Autodesk Inventor part; units mm, degrees
ref_plane "YZ Plane" through (0, 0, 0) normal (1, 0, 0) x (0, 1, 0)
ref_plane "XZ Plane" through (0, 0, 0) normal (0, 1, 0) x (-1, 0, 0)
ref_plane "XY Plane" through (0, 0, 0) normal (0, 0, 1) x (1, 0, 0)
sketch "Sketch1" plane through (0, 0, 0) normal (0, 0, 1) x (1, 0, 0)
  arc A0 (11.6951, -1.7956) -> (0, 0) centre (4.624, -8.8667) ccw
  line L0 (11.6951, -1.7956) -> (21.2005, -11.301)
  arc A1 (21.2005, -11.301) -> (22.9683, -12.0332) centre (22.9683, -9.5332) ccw
  line L1 (22.9683, -12.0332) -> (26.5038, -12.0332)
  arc A2 (26.5038, -12.0332) -> (29.0038, -9.5332) centre (26.5038, -9.5332) ccw
  line L2 (29.0038, -9.5332) -> (29.0038, -5.9977)
  arc A3 (29.0038, -5.9977) -> (28.2716, -4.2299) centre (26.5038, -5.9977) ccw
  line L3 (28.2716, -4.2299) -> (18.7662, 5.2754)
  arc A4 (16.9706, 16.9706) -> (18.7662, 5.2754) centre (25.8373, 12.3465) ccw
  arc A5 (16.9706, 16.9706) -> (16.9706, 53.963) centre (-18.4962, 35.4668) ccw
  arc A6 (18.7662, 65.6581) -> (16.9706, 53.963) centre (25.8373, 58.587) ccw
  line L4 (18.7662, 65.6581) -> (28.2716, 75.1635)
  arc A7 (28.2716, 75.1635) -> (29.0038, 76.9312) centre (26.5038, 76.9312) ccw
  line L5 (29.0038, 76.9312) -> (29.0038, 80.4668)
  arc A8 (29.0038, 80.4668) -> (26.5038, 82.9668) centre (26.5038, 80.4668) ccw
  line L6 (26.5038, 82.9668) -> (22.9683, 82.9668)
  arc A9 (22.9683, 82.9668) -> (21.2005, 82.2345) centre (22.9683, 80.4668) ccw
  line L7 (21.2005, 82.2345) -> (11.6951, 72.7291)
  arc A10 (0, 70.9335) -> (11.6951, 72.7291) centre (4.624, 79.8002) ccw
  arc A11 (0, 70.9335) -> (-36.9924, 70.9335) centre (-18.4962, 35.4668) ccw
  arc A12 (-48.6875, 72.7291) -> (-36.9924, 70.9335) centre (-41.6164, 79.8002) ccw
  line L8 (-48.6875, 72.7291) -> (-58.1929, 82.2345)
  arc A13 (-58.1929, 82.2345) -> (-59.9607, 82.9668) centre (-59.9607, 80.4668) ccw
  line L9 (-59.9607, 82.9668) -> (-63.4962, 82.9668)
  arc A14 (-63.4962, 82.9668) -> (-65.9962, 80.4668) centre (-63.4962, 80.4668) ccw
  line L10 (-65.9962, 80.4668) -> (-65.9962, 76.9312)
  arc A15 (-65.9962, 76.9312) -> (-65.264, 75.1635) centre (-63.4962, 76.9312) ccw
  line L11 (-65.264, 75.1635) -> (-55.7586, 65.6581)
  arc A16 (-53.9629, 53.963) -> (-55.7586, 65.6581) centre (-62.8296, 58.587) ccw
  arc A17 (-53.9629, 53.963) -> (-53.963, 16.9706) centre (-18.4962, 35.4668) ccw
  arc A18 (-55.7586, 5.2754) -> (-53.963, 16.9706) centre (-62.8296, 12.3465) ccw
  line L12 (-55.7586, 5.2754) -> (-65.264, -4.2299)
  arc A19 (-65.264, -4.2299) -> (-65.9962, -5.9977) centre (-63.4962, -5.9977) ccw
  line L13 (-65.9962, -5.9977) -> (-65.9962, -9.5332)
  arc A20 (-65.9962, -9.5332) -> (-63.4962, -12.0332) centre (-63.4962, -9.5332) ccw
  line L14 (-63.4962, -12.0332) -> (-59.9607, -12.0332)
  arc A21 (-59.9607, -12.0332) -> (-58.1929, -11.301) centre (-59.9607, -9.5332) ccw
  line L15 (-58.1929, -11.301) -> (-48.6875, -1.7956)
  arc A22 (-36.9924, 0) -> (-48.6875, -1.7956) centre (-41.6164, -8.8667) ccw
  arc A23 (-36.9924, 0) -> (-18.9962, -4.5301) centre (-18.4962, 35.4668) ccw
  arc A24 (-18.9962, -4.5301) -> (-17.9962, -4.5301) centre (-18.4962, -4.5332) ccw
  arc A25 (-17.9962, -4.5301) -> (0, 0) centre (-18.4962, 35.4668) ccw
  circle A26 centre (-49.9962, 3.9668) radius 3
  circle A27 centre (-49.9962, 66.9668) radius 3
  circle A28 centre (13.0038, 3.9668) radius 3
  circle A29 centre (13.0038, 66.9668) radius 3
  circle A30 centre (-18.4962, 35.4668) radius 36
extrude "Extrusion1" add sketch "Sketch1" along normal blind 400
sketch "Sketch2" plane through (0, 0, 400) normal (0, 0, 1) x (1, 0, 0)
  circle A0 centre (-18.4962, 35.4668) radius 36
  circle A1 centre (13.0038, 66.9668) radius 3
  circle A2 centre (13.0038, 3.9668) radius 3
  circle A3 centre (-49.9962, 66.9668) radius 3
  circle A4 centre (-49.9962, 3.9668) radius 3
  arc A5 (-17.9962, -4.5301) -> (0, 0) centre (-18.4962, 35.4668) ccw
  arc A6 (11.6951, -1.7956) -> (0, 0) centre (4.624, -8.8667) ccw
  line L0 (21.2005, -11.301) -> (11.6951, -1.7956)
  arc A7 (21.2005, -11.301) -> (22.9683, -12.0332) centre (22.9683, -9.5332) ccw
  line L1 (26.5038, -12.0332) -> (22.9683, -12.0332)
  arc A8 (26.5038, -12.0332) -> (29.0038, -9.5332) centre (26.5038, -9.5332) ccw
  line L2 (29.0038, -5.9977) -> (29.0038, -9.5332)
  arc A9 (29.0038, -5.9977) -> (28.2716, -4.2299) centre (26.5038, -5.9977) ccw
  line L3 (18.7662, 5.2754) -> (28.2716, -4.2299)
  arc A10 (16.9706, 16.9706) -> (18.7662, 5.2754) centre (25.8373, 12.3465) ccw
  arc A11 (16.9706, 16.9706) -> (16.9706, 53.963) centre (-18.4962, 35.4668) ccw
  arc A12 (18.7662, 65.6581) -> (16.9706, 53.963) centre (25.8373, 58.587) ccw
  line L4 (28.2716, 75.1635) -> (18.7662, 65.6581)
  arc A13 (28.2716, 75.1635) -> (29.0038, 76.9312) centre (26.5038, 76.9312) ccw
  line L5 (29.0038, 80.4668) -> (29.0038, 76.9312)
  arc A14 (29.0038, 80.4668) -> (26.5038, 82.9668) centre (26.5038, 80.4668) ccw
  line L6 (22.9683, 82.9668) -> (26.5038, 82.9668)
  arc A15 (22.9683, 82.9668) -> (21.2005, 82.2345) centre (22.9683, 80.4668) ccw
  line L7 (11.6951, 72.7291) -> (21.2005, 82.2345)
  arc A16 (0, 70.9335) -> (11.6951, 72.7291) centre (4.624, 79.8002) ccw
  arc A17 (0, 70.9335) -> (-36.9924, 70.9335) centre (-18.4962, 35.4668) ccw
  arc A18 (-48.6875, 72.7291) -> (-36.9924, 70.9335) centre (-41.6164, 79.8002) ccw
  line L8 (-58.1929, 82.2345) -> (-48.6875, 72.7291)
  arc A19 (-58.1929, 82.2345) -> (-59.9607, 82.9668) centre (-59.9607, 80.4668) ccw
  line L9 (-63.4962, 82.9668) -> (-59.9607, 82.9668)
  arc A20 (-63.4962, 82.9668) -> (-65.9962, 80.4668) centre (-63.4962, 80.4668) ccw
  line L10 (-65.9962, 76.9312) -> (-65.9962, 80.4668)
  arc A21 (-65.9962, 76.9312) -> (-65.264, 75.1635) centre (-63.4962, 76.9312) ccw
  line L11 (-55.7586, 65.6581) -> (-65.264, 75.1635)
  arc A22 (-53.9629, 53.963) -> (-55.7586, 65.6581) centre (-62.8296, 58.587) ccw
  arc A23 (-53.9629, 53.963) -> (-53.963, 16.9706) centre (-18.4962, 35.4668) ccw
  arc A24 (-55.7586, 5.2754) -> (-53.963, 16.9706) centre (-62.8296, 12.3465) ccw
  line L12 (-65.264, -4.2299) -> (-55.7586, 5.2754)
  arc A25 (-65.264, -4.2299) -> (-65.9962, -5.9977) centre (-63.4962, -5.9977) ccw
  line L13 (-65.9962, -9.5332) -> (-65.9962, -5.9977)
  arc A26 (-65.9962, -9.5332) -> (-63.4962, -12.0332) centre (-63.4962, -9.5332) ccw
  line L14 (-59.9607, -12.0332) -> (-63.4962, -12.0332)
  arc A27 (-59.9607, -12.0332) -> (-58.1929, -11.301) centre (-59.9607, -9.5332) ccw
  line L15 (-48.6875, -1.7956) -> (-58.1929, -11.301)
  arc A28 (-36.9924, 0) -> (-48.6875, -1.7956) centre (-41.6164, -8.8667) ccw
  arc A29 (-36.9924, 0) -> (-18.9962, -4.5301) centre (-18.4962, 35.4668) ccw
  arc A30 (-18.9962, -4.5301) -> (-17.9962, -4.5301) centre (-18.4962, -4.5332) ccw
extrude "Extrusion2" cut sketch "Sketch2" against normal blind 250
sketch "Sketch3" plane through (-63.4962, -12.0332, 0) normal (0, -1, 0) x (1, 0, 0)
  line L0 (0, 0) -> (0, 150)
  line L1 (-3.0046, 150) -> (99.6718, 150)
  line L2 (99.6718, 150) -> (99.6718, 100)
  line L3 (99.6718, 100) -> (-3.0046, 100)
  line L4 (-3.0046, 100) -> (-3.0046, 150)
  point P0 (63.4962, 0)
  dimension "d4" = 50
  dimension "d5" = 102.6763
  dimension "d6" = 3.0046
extrude "Extrusion3" cut sketch "Sketch3" against normal blind 95
properties part number "X95_100mm"
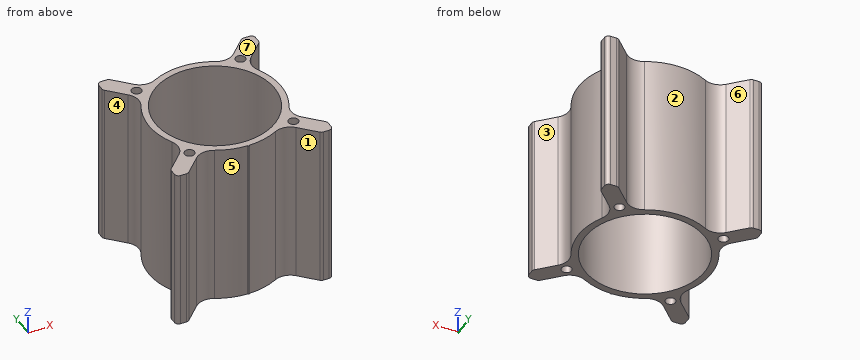
Geometry check sheet. Reference: the model listing, model coordinates, mm. Face numbers are marked on the shaded views. A direction names the side the tool comes from. Round coordinates to 2 decimals unless told otherwise and drop trailing zeros. Write each loop counter-clockwise with the first axis right and the second up, starting at its lowest first coordinate (ties: lowest second). Pieces come first, ordered by that corner, then holes.
Item 1: Material ranges on line 1 along Y through (x, z) = (18, 28); line 2 along Y through (x, z) = (-20, 13); line 3 along Y through (x, z) = (9.5, 53.5), recorded low to high.
Determined:
line 1: y = -8.1 to 6.14, 19.1 to 51.84, 64.8 to 79.03
line 2: y = -4.5 to -0.5, 71.44 to 75.44
line 3: y = -0.14 to 12.83, 58.1 to 71.07
Item 2: Access from +Z, -Z, +X, -X, +Y, -Y to the whole of each face (thin tool, end or side, straight path). Record for the marked faces 5, 6 and 7.
Determined:
face 5: +Z, -Z, -Y
face 6: +Z, -Z, +Y
face 7: +Z, +X, -X, +Y, -Y
Item 3: Section check B-B (y = 47.5). Record the boundary of the cut face in (x, z), plus the area to 3 significant figures.
Determined:
outline: (-56.64, 0) - (-52.43, 0) - (-52.43, 100) - (-56.64, 100) - close; (15.43, 0) - (19.65, 0) - (19.65, 100) - (15.43, 100) - close
area: 844 mm2
Item 4: Go/stop test with flat-tipped pins: pin 1 Ø1.5 at (y, z) = (19, 30) entering from -X; pin 2 Ø5.5 at (x, y) = (13, 3.97) entering from -Z; pin 3 Ø5 at (x, z) = (-38, 21) entering from +Y; pin 4 Ø6 at (y, z) = (30.5, 81.5) entering from -X. Record where each tip stops, or that it passes through.
Determined:
pin 1: stops at x = -55.28
pin 2: passes through
pin 3: stops at y = 71.67
pin 4: stops at x = -58.45
Item 5: Mould release check, pull along X, two halves, no side actions. Record for the marked faces 1, 2, 3 and 4: +X half, -X half, draft (parallel to the pull), parting line (faces both ways), or undercut.
Determined:
face 1: undercut
face 2: undercut
face 3: +X half
face 4: -X half
Item 6: Section check A-A (x = -41). Record the boundary of the cut face in (y, z), plus the area to 3 significant figures.
Determined:
outline: (1.11, 0) - (7.37, 0) - (7.37, 100) - (1.11, 100) - close; (63.57, 0) - (69.82, 0) - (69.82, 100) - (63.57, 100) - close
area: 1,250 mm2
Item 7: Section check C-C (z = 52). Give the number of separate pieces and of enclosed holes in the cut face, plus the area to 3 significant figures.
Determined:
separate pieces: 1
enclosed holes: 5
area: 1,920 mm2
